Check sheet for the drawn part. Datum: minimum x, y, z corner. Units: mm. A direction names the side the tool comes from. Coordinates: 2 decimals unless noted, no trailing zeros. Order: outer loops, then holes, each group sorted by start corner. A loop starts at its lowest first (then second) coordinate and runs counter-clockwise, first axis right, second up. Notation, with made-up numbers: (82, 55) - (97, 55) arc R31 cw to (97, 80) - close; hole circle Ø1 at (-9, -17.75). An arc over 180 degrees is marked (long way). Put each result on its own line as item: value.
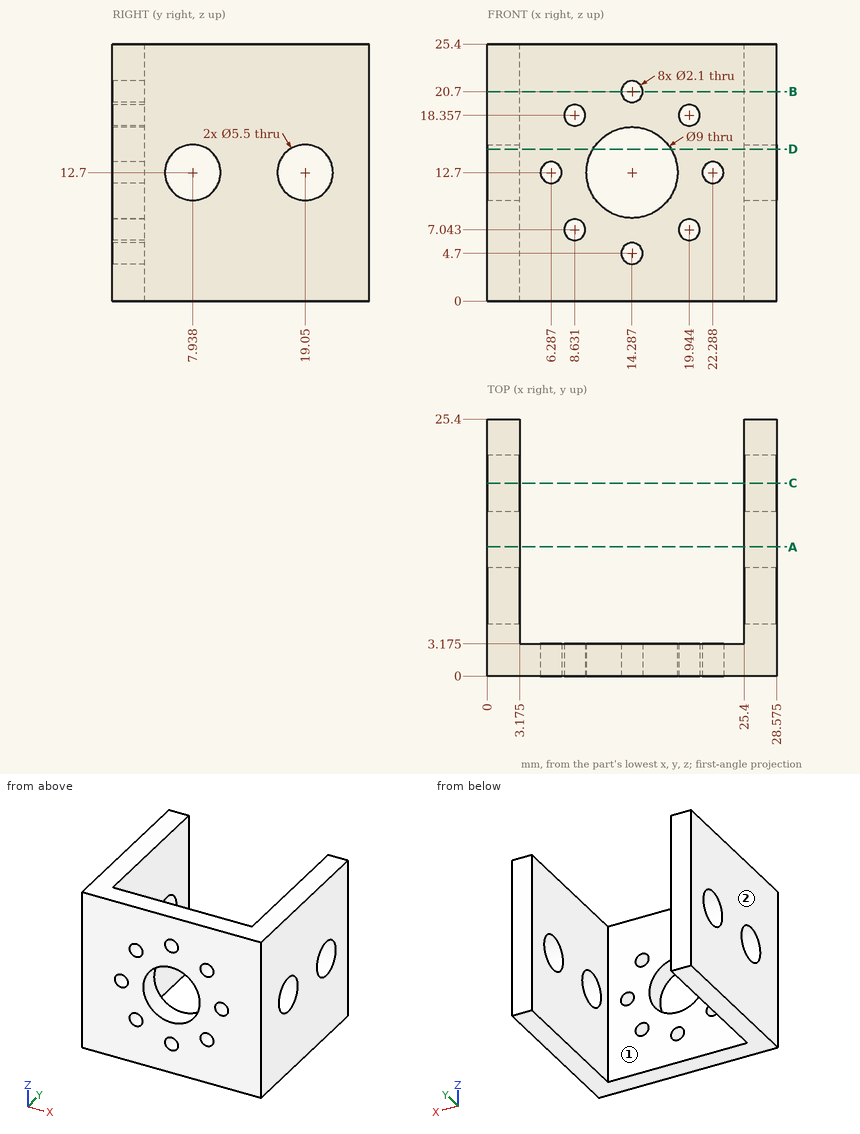
Q1. Depth check by flat-ended pin: pin 1 Ø10.5 at (x, z) = (14.29, 12.7) entering from -Y; pin 2 Ø4.5 at (y, z) = (7.94, 12.7) entering from -X; pin 3 Ø3.5 at (x, z) = (6.29, 12.7) entering from +Y (1 decimal). Enter the tip coordinate at first touch or a pass-through.
Answer block:
pin 1: stops at y = 0
pin 2: passes through
pin 3: stops at y = 3.2
Q2. Thickness scan on L1, parallel to Y at x = 26.25, z = 12.5 (1 decimal); L2, parallel to X at y = 7.5, z = 20 (1 decimal); L3, parallel to X at y = 2.25, z = 7.5 (1 decimal). Record the ranges inside material, lowest first. Write a range as [from, to].
Answer block:
L1: y = [0, 5.2], [10.7, 16.3], [21.8, 25.4]
L2: x = [0, 3.2], [25.4, 28.6]
L3: x = [0, 7.7], [9.6, 19], [20.9, 28.6]
Q3. Section check A-A on y = 12.75. Record the boundary of the cut face in (x, z) (1 decimal).
Answer block:
outline: (0, 0) - (3.2, 0) - (3.2, 25.4) - (0, 25.4) - close; (25.4, 0) - (28.6, 0) - (28.6, 25.4) - (25.4, 25.4) - close
Q4. Section check C-C on y = 19.05. State how many separate pieces and enclosed holes the cut face has, then the cut area to 3 significant figures.
Answer block:
separate pieces: 4
enclosed holes: 0
area: 126 mm^2
Q5. Section check D-D on z = 15. Record the boundary of the cut face in (x, y) (1 decimal).
Answer block:
outline: (0, 0) - (10.4, 0) - (10.4, 3.2) - (3.2, 3.2) - (3.2, 6.4) - (0, 6.4) - close; (0, 9.4) - (3.2, 9.4) - (3.2, 17.5) - (0, 17.5) - close; (0, 20.6) - (3.2, 20.6) - (3.2, 25.4) - (0, 25.4) - close; (18.2, 0) - (28.6, 0) - (28.6, 6.4) - (25.4, 6.4) - (25.4, 3.2) - (18.2, 3.2) - close; (25.4, 9.4) - (28.6, 9.4) - (28.6, 17.5) - (25.4, 17.5) - close; (25.4, 20.6) - (28.6, 20.6) - (28.6, 25.4) - (25.4, 25.4) - close
Q6. Section check B-B on z = 20.7. Record the boundary of the cut face in (x, y) (1 decimal).
Answer block:
outline: (0, 0) - (13.2, 0) - (13.2, 3.2) - (3.2, 3.2) - (3.2, 25.4) - (0, 25.4) - close; (15.3, 0) - (28.6, 0) - (28.6, 25.4) - (25.4, 25.4) - (25.4, 3.2) - (15.3, 3.2) - close
Q7. Access from +Z, -Z, +X, -X, +Y, -Y to the whole of each face (thin tool, end or side, straight path). Record for the marked faces 1 and 2.
Answer block:
face 1: +Z, -Z, +Y
face 2: +Z, -Z, -X, +Y, -Y
